Autodesk Inventor part; units mm, degrees
ref_plane "YZ Plane" through (0, 0, 0) normal (1, 0, 0) x (0, 1, 0)
ref_plane "XZ Plane" through (0, 0, 0) normal (0, 1, 0) x (-1, 0, 0)
ref_plane "XY Plane" through (0, 0, 0) normal (0, 0, 1) x (1, 0, 0)
sketch "Sketch1" plane through (0, 0, 0) normal (1, 0, 0) x (0, 1, 0)
  arc A0 (0.7409, -6.9281) -> (1.6287, -5.6125) centre (1.1834, -6.2693) ccw
  line L0 (1.6287, -5.6125) -> (1.2582, -6.1591)
  line L1 (0.7409, -6.9281) -> (1.1092, -6.3799) construction
  line L2 (2.519, -4.2812) -> (2.1507, -4.8294) construction
  arc A1 (1.1092, -6.3799) -> (1.2582, -6.1591) centre (1.1834, -6.2693) ccw
  arc A2 (2.1507, -4.8294) -> (1.1092, -6.3799) centre (1.63, -5.6046) ccw
  arc A3 (2.1507, -4.8294) -> (12.3205, -4.2899) centre (6.8767, 2.206) ccw
  arc A4 (2.519, -4.2812) -> (11.8963, -3.7838) centre (6.8767, 2.206) ccw
  arc A5 (12.3205, -4.2899) -> (12.9142, -3.0177) centre (11.2543, -3.0177) ccw
  arc A6 (11.8963, -3.7838) -> (12.2538, -3.0177) centre (11.2543, -3.0177) ccw
  line L3 (11.8963, -3.7838) -> (12.3205, -4.2899) construction
  line L4 (12.2538, -3.0177) -> (12.9142, -3.0177) construction
  arc A7 (12.2538, -3.0177) -> (10.7251, -3.0177) centre (11.4895, -3.0177) ccw
  line L5 (10.7251, -3.0177) -> (10.0647, -3.0177)
  arc A8 (12.9142, -3.0177) -> (10.0647, -3.0177) centre (11.4895, -3.0177) ccw
  line L6 (0.0665, -5.2922) -> (0.0665, -5.917)
  arc A9 (2.519, -4.2812) -> (0.0665, -5.2922) centre (1.63, -5.6046) ccw
  arc A10 (0.0665, -5.917) -> (0.7409, -6.9281) centre (1.63, -5.6046) ccw
  point P0 (0, 0)
  point P1 (12.584, -3.0177)
  dimension "d10" = 0.6604
  dimension "d11" = 0.6604
  dimension "d12" = 0.6604
  dimension "d15" = 0.6604
extrude "leg" add sketch "Sketch1" along normal mid plane 0.6604
pattern_circular "Circular Pattern1" count 3 over 360 about axis through (0, -10, 0) along (0, 1, 0) of "leg"
sketch "Sketch2" plane through (0, 0, 0) normal (1, 0, 0) x (0, 1, 0)
  arc A0 (11.8963, -3.7838) -> (12.2538, -3.0177) centre (11.2543, -3.0177) ccw
  arc A1 (12.3205, -4.2899) -> (12.9142, -3.0177) centre (11.2543, -3.0177) ccw
  arc A2 (11.8963, -3.7838) -> (12.2538, -3.0177) centre (11.2543, -3.0177) ccw
  line L0 (12.2538, -3.0177) -> (12.9142, -3.0177)
  line L1 (12.584, -3.0177) -> (13.2952, -3.0177) construction
  line L2 (13.2952, -3.0177) -> (13.2952, 0.0049)
  line L3 (13.2952, 0.0049) -> (12.584, 0.0049)
  line L4 (12.584, 0.0049) -> (12.584, -3.0177)
  line L5 (13.2952, -3.0177) -> (13.2952, -8.0977)
  line L6 (13.2952, -8.0977) -> (12.584, -8.0977)
  line L7 (12.584, -8.0977) -> (12.584, -3.0177)
  point P0 (0, 0)
  dimension "d21" = 0.7112
  dimension "d22" = 3.0226
  dimension "d23" = 5.08
revolve "Revolution1" add sketch "Sketch2" angle 360 about axis through (0, 13.2952, 0.0049) along (0, -1, 0)
properties part number "table round"
Verification items for the finished model (mm, model axes). A direction names the side the tool comes from. Round coordinates to 2 decimals unless told otherwise and drop trailing zeros. Write each loop counter-clockwise with the first axis right and the second up, starting at its lowest first coordinate (ties: lowest second). Pieces come first, ordered by that corner, then holes.
(1) Section check C-C (z = 0). Enter the section's corners in (x, y), plus the area to 3 significant figures.
Returned:
outline: (-8.1, 12.58) - (8.1, 12.58) - (8.1, 13.3) - (-8.1, 13.3) - close
area: 11.5 mm2
(2) Mould release check, pull along Y, two halves, no side actions. Record for faces 1 (the flat face through (-4.8, 0.066, 2.8)), 2 (the flat face through (5.306, 6.296, 2.682)), 3 (the cylindrical face through (-1.458, 10.982, 0.847)): pulls with the +Y half, pulls with the -Y half, needs draft (parallel to the pull), parting line crosses it, or undercut.
Returned:
face 1: pulls with the -Y half
face 2: needs draft
face 3: undercut
(3) Section check D-D (y = 8). Enter the section's corners in (x, z).
Returned:
outline: (-5.53, 2.81) - (-4.95, 2.48) - (-4.62, 3.05) - (-5.2, 3.38) - close; (-0.33, -6.19) - (0.33, -6.19) - (0.33, -5.53) - (-0.33, -5.53) - close; (4.62, 3.05) - (4.95, 2.48) - (5.53, 2.81) - (5.2, 3.38) - close
(4) Section check A-A (y = 9.5). Enter the section's corners in (x, z), plus the area to 3 significant figures.
Returned:
outline: (-5.23, 2.64) - (-4.63, 2.29) - (-4.3, 2.86) - (-4.9, 3.21) - close; (-0.33, -5.85) - (0.33, -5.85) - (0.33, -5.16) - (-0.33, -5.16) - close; (4.3, 2.86) - (4.63, 2.29) - (5.23, 2.64) - (4.9, 3.21) - close
area: 1.38 mm2
(5) Depth check by flat-ended pin: pin 1 Ø5 at (x, y) = (-4, 11.5) entering from +Z; pin 2 Ø1.6 at (y, z) = (4.5, -4.5) entering from +X; pin 3 Ø1 at (x, y) = (0.5, 10) entering from +Z. Enter the tip coordinate at first touch or a pass-through.
Returned:
pin 1: stops at z = 7.92
pin 2: stops at x = 0.33
pin 3: stops at z = -2.02
(6) Section check B-B (x = 0). Enter the section's corners in (y, z), plus the area to 3 significant figures.
Returned:
outline: (0.07, -5.92) arc R1.59 ccw to (0.74, -6.93) arc R0.79 ccw to (1.63, -5.61) - (1.26, -6.16) arc R0.13 cw to (1.11, -6.38) arc R0.93 cw to (2.15, -4.83) arc R8.48 ccw to (12.32, -4.29) arc R1.66 ccw to (12.58, -4.01) - (12.58, -8.1) - (13.3, -8.1) - (13.3, 8.11) - (12.58, 8.11) - (12.58, -2.11) arc R1.42 ccw to (10.06, -3.02) - (10.73, -3.02) arc R0.76 cw to (12.25, -3.02) arc R1 cw to (11.9, -3.78) arc R7.82 cw to (2.52, -4.28) arc R1.59 ccw to (0.07, -5.29) - close
area: 24.6 mm2
(7) Material ranges on line 1 (Y direction, x = 3.25, z = -2.5); line 2 (X direction, y = 5.75, z = -6); line 3 (Y direction, x = 4.5, z = 2.5), recorded low to high.
Returned:
line 1: y = 12.58 to 13.3
line 2: x = -0.33 to 0.33
line 3: y = 0.1 to 0.82, 2.66 to 4.23, 9.52 to 11.09, 12.58 to 13.3
(8) Access from +Z, -Z, +X, -X, +Y, -Y to the whole of each face (thin tool, end or side, straight path). Record for faces 4 (the cylindrical face through (-0.005, 7.361, -5.594)), 5 (the flat face through (0.33, 6, -6)), 6 (the flat face through (-0.33, 6, -6)).
Returned:
face 4: +X, -X
face 5: +Z, -Z, +X, -Y
face 6: +Z, -Z, -X, -Y
